from build123d import *

# Parameters (mm, degrees)
SKETCH1_W           = 40
SKETCH1_H           = 50
BOSS_EXTRUDE1_DEPTH = 5
CUT_EXTRUDE1_DEPTH  = 169.198858526
FILLET1_R           = 3
SKETCH3_R           = 1.5875
CUT_EXTRUDE2_DEPTH  = 169.198858526
CUT_EXTRUDE3_DEPTH  = 169.198858526
CUT_EXTRUDE5_DEPTH  = 5
SKETCH7_R           = 2.5
CUT_EXTRUDE6_DEPTH  = 5
SKETCH8_W           = 65
SKETCH8_H           = 22.934618833
CUT_EXTRUDE7_DEPTH  = 5


with BuildPart() as part:
    # Sketch1 → Boss-Extrude1 (new body)
    with BuildSketch(Plane.XY):
        with BuildLine():
            Line((149.732146976, -33.800912799), (144.732146976, -33.800912799))
            Line((144.732146976, -33.800912799), (144.732146976, 46.199087201))
            Line((144.732146976, 46.199087201), (149.732146976, 46.199087201))
            Line((149.732146976, 46.199087201), (149.732146976, 54.598220465))
            Line((149.732146976, 54.598220465), (129.732146976, 74.598220465))
            Line((129.732146976, 74.598220465), (-130.267853024, 74.598220465))
            Line((-130.267853024, 74.598220465), (-150.267853024, 54.598220465))
            Line((-150.267853024, 54.598220465), (-150.267853024, 46.199087201))
            Line((-150.267853024, 46.199087201), (-145.267853024, 46.199087201))
            Line((-145.267853024, 46.199087201), (-145.267853024, -33.800912799))
            Line((-145.267853024, -33.800912799), (-150.267853024, -33.800912799))
            Line((-150.267853024, -33.800912799), (-150.267853024, -55.401779535))
            Line((-150.267853024, -55.401779535), (-130.267853024, -75.401779535))
            Line((-130.267853024, -75.401779535), (-83.434100927, -75.401779535))
            Line((-83.434100927, -75.401779535), (-50.267853024, -42.235531632))
            Line((-50.267853024, -42.235531632), (-28.267853024, -42.235531632))
            ThreePointArc((-28.267853024, -42.235531632), (-26.14653268, -41.356851975), (-25.267853024, -39.235531632))
            Line((-25.267853024, -39.235531632), (-25.267853024, 1.264468368))
            ThreePointArc((-25.267853024, 1.264468368), (-24.389173367, 3.385788712), (-22.267853024, 4.264468368))
            Line((-22.267853024, 4.264468368), (21.732146976, 4.264468368))
            ThreePointArc((21.732146976, 4.264468368), (23.85346732, 3.385788712), (24.732146976, 1.264468368))
            Line((24.732146976, 1.264468368), (24.732146976, -39.235531632))
            ThreePointArc((24.732146976, -39.235531632), (25.610826633, -41.356851975), (27.732146976, -42.235531632))
            Line((27.732146976, -42.235531632), (49.732146976, -42.235531632))
            Line((49.732146976, -42.235531632), (82.89839488, -75.401779535))
            Line((82.89839488, -75.401779535), (129.732146976, -75.401779535))
            Line((129.732146976, -75.401779535), (149.732146976, -55.401779535))
            Line((149.732146976, -55.401779535), (149.732146976, -33.800912799))
        make_face()
        with Locations((-52.767853024, 6.199087201)):
            Rectangle(SKETCH1_W, SKETCH1_H, mode=Mode.SUBTRACT)
        with Locations((52.232146976, 6.199087201)):
            Rectangle(SKETCH1_W, SKETCH1_H, mode=Mode.SUBTRACT)
    extrude(amount=BOSS_EXTRUDE1_DEPTH)

    # Sketch2 → Cut-Extrude1 (cut, through all)
    with BuildSketch(Plane.XY.offset(5)):
        with BuildLine():
            ThreePointArc((21.732146976, 4.264468368), (23.85346732, 3.385788712), (24.732146976, 1.264468368))
            Line((24.732146976, 1.264468368), (24.732146976, -39.235531632))
            ThreePointArc((24.732146976, -39.235531632), (25.610826633, -41.356851975), (27.732146976, -42.235531632))
            Line((27.732146976, -42.235531632), (28.732146976, -42.235531632))
            Line((28.732146976, -42.235531632), (28.732146976, -38.362548286))
            Line((28.732146976, -38.362548286), (28.732146976, 1.264468368))
            ThreePointArc((28.732146976, 1.264468368), (26.681894445, 6.214215837), (21.732146976, 8.264468368))
            Line((21.732146976, 8.264468368), (-22.267853024, 8.264468368))
            ThreePointArc((-22.267853024, 8.264468368), (-27.217600492, 6.214215837), (-29.267853024, 1.264468368))
            Line((-29.267853024, 1.264468368), (-29.267853024, -38.362548286))
            Line((-29.267853024, -38.362548286), (-29.267853024, -42.235531632))
            Line((-29.267853024, -42.235531632), (-28.267853024, -42.235531632))
            ThreePointArc((-28.267853024, -42.235531632), (-26.14653268, -41.356851975), (-25.267853024, -39.235531632))
            Line((-25.267853024, -39.235531632), (-25.267853024, 1.264468368))
            ThreePointArc((-25.267853024, 1.264468368), (-24.389173367, 3.385788712), (-22.267853024, 4.264468368))
            Line((-22.267853024, 4.264468368), (21.732146976, 4.264468368))
        make_face()
    extrude(amount=-CUT_EXTRUDE1_DEPTH, mode=Mode.SUBTRACT)

    # Fillet1
    fillet1_edges = [part.edges().sort_by_distance(p)[0] for p in [
        (28.732146976, -42.235531632, 2.5),
        (-29.267853024, -42.235531632, 2.5),
    ]]
    fillet(fillet1_edges, radius=FILLET1_R)

    # Sketch3 → Cut-Extrude2 (cut, through all)
    with BuildSketch(Plane.XY.offset(5)):
        with Locations((-78.605353024, -9.421912799)):
            Circle(SKETCH3_R)
        with Locations((-78.605353024, 21.820087201)):
            Circle(SKETCH3_R)
        with Locations((-84.955353024, -9.421912799)):
            Circle(SKETCH3_R)
        with Locations((-84.955353024, 21.820087201)):
            Circle(SKETCH3_R)
        with Locations((-91.305353024, -9.421912799)):
            Circle(SKETCH3_R)
        with Locations((-91.305353024, 21.820087201)):
            Circle(SKETCH3_R)
        with Locations((-97.655353024, -9.421912799)):
            Circle(SKETCH3_R)
        with Locations((-97.655353024, 21.820087201)):
            Circle(SKETCH3_R)
        with Locations((-104.005353024, -9.421912799)):
            Circle(SKETCH3_R)
        with Locations((-104.005353024, 21.820087201)):
            Circle(SKETCH3_R)
        with Locations((-110.355353024, -9.421912799)):
            Circle(SKETCH3_R)
        with Locations((-110.355353024, 21.820087201)):
            Circle(SKETCH3_R)
        with Locations((-116.705353024, -9.421912799)):
            Circle(SKETCH3_R)
        with Locations((-116.705353024, 21.820087201)):
            Circle(SKETCH3_R)
        with Locations((-123.055353024, -9.421912799)):
            Circle(SKETCH3_R)
        with Locations((-123.055353024, 21.820087201)):
            Circle(SKETCH3_R)
        with Locations((-129.405353024, -9.421912799)):
            Circle(SKETCH3_R)
        with Locations((-129.405353024, 21.820087201)):
            Circle(SKETCH3_R)
        with Locations((-135.755353024, -9.421912799)):
            Circle(SKETCH3_R)
        with Locations((-135.755353024, 21.820087201)):
            Circle(SKETCH3_R)
        with Locations(Location((135.219646976, 21.820087201, 0), (0, 0, 180))):
            Circle(SKETCH3_R)
        with Locations(Location((135.219646976, -9.421912799, 0), (0, 0, 180))):
            Circle(SKETCH3_R)
        with Locations(Location((128.869646976, 21.820087201, 0), (0, 0, 180))):
            Circle(SKETCH3_R)
        with Locations(Location((128.869646976, -9.421912799, 0), (0, 0, 180))):
            Circle(SKETCH3_R)
        with Locations(Location((122.519646976, 21.820087201, 0), (0, 0, 180))):
            Circle(SKETCH3_R)
        with Locations(Location((122.519646976, -9.421912799, 0), (0, 0, 180))):
            Circle(SKETCH3_R)
        with Locations(Location((116.169646976, 21.820087201, 0), (0, 0, 180))):
            Circle(SKETCH3_R)
        with Locations(Location((116.169646976, -9.421912799, 0), (0, 0, 180))):
            Circle(SKETCH3_R)
        with Locations(Location((109.819646976, 21.820087201, 0), (0, 0, 180))):
            Circle(SKETCH3_R)
        with Locations(Location((109.819646976, -9.421912799, 0), (0, 0, 180))):
            Circle(SKETCH3_R)
        with Locations(Location((103.469646976, 21.820087201, 0), (0, 0, 180))):
            Circle(SKETCH3_R)
        with Locations(Location((103.469646976, -9.421912799, 0), (0, 0, 180))):
            Circle(SKETCH3_R)
        with Locations(Location((97.119646976, 21.820087201, 0), (0, 0, 180))):
            Circle(SKETCH3_R)
        with Locations(Location((97.119646976, -9.421912799, 0), (0, 0, 180))):
            Circle(SKETCH3_R)
        with Locations(Location((90.769646976, 21.820087201, 0), (0, 0, 180))):
            Circle(SKETCH3_R)
        with Locations(Location((90.769646976, -9.421912799, 0), (0, 0, 180))):
            Circle(SKETCH3_R)
        with Locations(Location((84.419646976, 21.820087201, 0), (0, 0, 180))):
            Circle(SKETCH3_R)
        with Locations(Location((84.419646976, -9.421912799, 0), (0, 0, 180))):
            Circle(SKETCH3_R)
        with Locations(Location((78.069646976, 21.820087201, 0), (0, 0, 180))):
            Circle(SKETCH3_R)
        with Locations(Location((78.069646976, -9.421912799, 0), (0, 0, 180))):
            Circle(SKETCH3_R)
    extrude(amount=-CUT_EXTRUDE2_DEPTH, mode=Mode.SUBTRACT)

    # Sketch4 → Cut-Extrude3 (cut, through all)
    with BuildSketch(Plane.XY.offset(5)):
        with BuildLine():
            Line((-41.267853024, -42.235531632), (-41.267853024, -18.800912799))
            Line((-41.267853024, -18.800912799), (-32.767853024, -18.800912799))
            Line((-32.767853024, -18.800912799), (-32.767853024, 8.264468368))
            Line((-32.767853024, 8.264468368), (-22.267853024, 8.264468368))
            ThreePointArc((-22.267853024, 8.264468368), (-27.217600492, 6.214215837), (-29.267853024, 1.264468368))
            Line((-29.267853024, 1.264468368), (-29.267853024, -39.235531632))
            ThreePointArc((-29.267853024, -39.235531632), (-30.14653268, -41.356851975), (-32.267853024, -42.235531632))
            Line((-32.267853024, -42.235531632), (-41.267853024, -42.235531632))
        make_face()
        with BuildLine():
            Line((21.732146976, 8.264468368), (32.232146976, 8.264468368))
            Line((32.232146976, 8.264468368), (32.232146976, -18.800912799))
            Line((32.232146976, -18.800912799), (40.732146976, -18.800912799))
            Line((40.732146976, -18.800912799), (40.732146976, -42.235531632))
            Line((40.732146976, -42.235531632), (31.732146976, -42.235531632))
            ThreePointArc((31.732146976, -42.235531632), (29.610826633, -41.356851975), (28.732146976, -39.235531632))
            Line((28.732146976, -39.235531632), (28.732146976, 1.264468368))
            ThreePointArc((28.732146976, 1.264468368), (26.681894445, 6.214215837), (21.732146976, 8.264468368))
        make_face()
    extrude(amount=-CUT_EXTRUDE3_DEPTH, mode=Mode.SUBTRACT)

    # Sketch6 → Cut-Extrude5 (cut)
    with BuildSketch(Plane.XY.offset(5)):
        Polygon((-102.767853024, 74.598220465), (-102.767853024, 69.598220465), (-94.867853024, 69.598220465), (-94.867853024, 64.598220465), (-97.767853024, 64.598220465), (-97.767853024, 54.598220465), (-87.767853024, 54.598220465), (-87.767853024, 64.598220465), (-90.667853024, 64.598220465), (-90.667853024, 69.598220465), (-82.767853024, 69.598220465), (-82.767853024, 74.598220465), align=None)
        Polygon((-116.850976975, -75.401779535), (-116.850976975, -70.401779535), (-108.950976975, -70.401779535), (-108.950976975, -65.401779535), (-111.850976975, -65.401779535), (-111.850976975, -55.401779535), (-101.850976975, -55.401779535), (-101.850976975, -65.401779535), (-104.750976975, -65.401779535), (-104.750976975, -70.401779535), (-96.850976975, -70.401779535), (-96.850976975, -75.401779535), align=None)
        Polygon((104.215270928, -70.401779535), (96.315270928, -70.401779535), (96.315270928, -75.401779535), (116.315270928, -75.401779535), (116.315270928, -70.401779535), (108.415270928, -70.401779535), (108.415270928, -65.401779535), (111.315270928, -65.401779535), (111.315270928, -55.401779535), (101.315270928, -55.401779535), (101.315270928, -65.401779535), (104.215270928, -65.401779535), align=None)
        Polygon((90.132146976, 69.598220465), (82.232146976, 69.598220465), (82.232146976, 74.598220465), (102.232146976, 74.598220465), (102.232146976, 69.598220465), (94.332146976, 69.598220465), (94.332146976, 64.598220465), (97.232146976, 64.598220465), (97.232146976, 54.598220465), (87.232146976, 54.598220465), (87.232146976, 64.598220465), (90.132146976, 64.598220465), align=None)
    extrude(amount=-CUT_EXTRUDE5_DEPTH, mode=Mode.SUBTRACT)

    # Sketch7 → Cut-Extrude6 (cut)
    with BuildSketch(Plane.XY.offset(5)):
        with Locations((-133.267853024, -19.300912799)):
            Circle(SKETCH7_R)
        with Locations((-133.267853024, 31.699087201)):
            Circle(SKETCH7_R)
        with Locations((132.732146976, -19.300912799)):
            Circle(SKETCH7_R)
        with Locations((132.732146976, 31.699087201)):
            Circle(SKETCH7_R)
    extrude(amount=-CUT_EXTRUDE6_DEPTH, mode=Mode.SUBTRACT)

    # Sketch8 → Cut-Extrude7 (cut)
    with BuildSketch(Plane.XY.offset(5)):
        with Locations((-0.267853024, 19.731777785)):
            Rectangle(SKETCH8_W, SKETCH8_H)
    extrude(amount=-CUT_EXTRUDE7_DEPTH, mode=Mode.SUBTRACT)


solid = part.part
Build history of the part. All positions in model axes, mm. Round coordinates to 2 decimals unless told otherwise and drop trailing zeros. Write each loop counter-clockwise with the first axis right and the second up, starting at its lowest first coordinate (ties: lowest second). Pieces come first, ordered by that corner, then holes. Notation, with made-up numbers: (54, 43) -> (79, 43) arc R22 cw to (79, 64) -> close; hole circle Ø6 at (75, 46.25). An arc over 180 degrees is marked (long way). Use one line per item in the form item = value.
Q1. Band-saw the part on A-A, the plane y = 11. Write the cut outline in (x, z).
Conclusion:
outline = (-145.27, 0) -> (-72.77, 0) -> (-72.77, 5) -> (-145.27, 5) -> close; (72.23, 0) -> (144.73, 0) -> (144.73, 5) -> (72.23, 5) -> close
Q2. Drop flat-ended pins along their axis: P1, Ø1, axis at y = -5.5, z = 2, coming from the -X side; P2, Ø1.5, axis at y = -59, z = 2, coming from the +X side; P3, Ø2.5, axis at x = 93.5, z = 3, coming from the +Y side. Give the stop position or say it passes through.
Conclusion:
P1 = -145.27
P2 = 146.88
P3 = 69.6
Q3. Band-saw the part on C-C, the plane y = 60.5. Write the cut outline in (x, z), then the cut area to 3 significant figures.
Conclusion:
outline = (-144.37, 0) -> (-97.77, 0) -> (-97.77, 5) -> (-144.37, 5) -> close; (-87.77, 0) -> (87.23, 0) -> (87.23, 5) -> (-87.77, 5) -> close; (97.23, 0) -> (143.83, 0) -> (143.83, 5) -> (97.23, 5) -> close
area = 1,340 mm²
Q4. Two-plate mould, pull along X, no slides. Class faces 1 (the flat face through (-140.41, -65.26, 2.46)), 2 (the flat face through (-67.08, -59.05, 2.46)), 3 (the flat face through (66.083, -58.586, 2.465)), 4 (the flat face through (139.592, -65.542, 2.465)): released by +X, released by -X, zero draft, split by the parting line, or undercut.
Conclusion:
face_1 = released by -X
face_2 = undercut
face_3 = undercut
face_4 = released by +X
Q5. Drill centre lines: L1, parallel to X at y = 67.5, z = 2.4; L2, parallel to Y at x = -47, z = 3; L3, parallel to X at y = -28.5, z = 0.45. Where is each one in solid material? Low to high.
Conclusion:
L1 = -137.37 to -94.87, -90.67 to 90.13, 94.33 to 136.83
L2 = -42.24 to -18.8, 31.2 to 74.6
L3 = -145.27 to -41.27, 40.73 to 144.73
Q6. Band-saw the part on B-B, the plane x = -62. Write the cut outline in (y, z), then the cut area to 3 significant figures.
Conclusion:
outline = (-53.97, 0) -> (-18.8, 0) -> (-18.8, 5) -> (-53.97, 5) -> close; (31.2, 0) -> (74.6, 0) -> (74.6, 5) -> (31.2, 5) -> close
area = 393 mm²
Q7. Band-saw the part on D-D, the plane z = 3. State how many separate pieces and enclosed holes the cut face has, then the cut area to 3 significant figures.
Conclusion:
separate_pieces = 1
enclosed_holes = 44
area = 28,500 mm²
